CAD build for the part. Positions are in the model's coordinates, mm. Face numbers are marked on the shaded views. A direction names the side the tool comes from. Coordinates: 2 decimals unless noted, no trailing zeros. Order: outer loops, then holes, each group sorted by start corner. A loop starts at its lowest first (then second) coordinate and runs counter-clockwise, first axis right, second up. Notation, with made-up numbers: (89, 55) - (135, 55) arc R19 ccw to (135, 75) - close; hole circle Ø1 at (36.25, 0). An arc over 180 degrees is marked (long way). Write each question's results on one line, items separated by ' | '. Start each with the question number.
Q1. Pull direction Z, two halves, no side cores. Call the marked faces 1, 2 and 3: released by +Z, released by -Z, zero draft, split by the parting line, or undercut.
Q2. Band-saw the part on B-B, the plane z = -31. Write the cut outline in (x, y), then the cut area to 3 significant figures.
Q3. Band-saw the part on D-D, the plane z = 47.5. Write the cut outline in (x, y), then the cut area to 3 significant figures.
Q4. Band-saw the part on A-A, the plane z = -3. Write the cut outline in (x, y), then the cut area to 3 significant figures.
Q5. Wall check: probe 1 along X at (y, z) = (30, -5); probe 2 along X at (y, z) = (32, -34.5); probe 3 along X at (y, z) = (32, -73). Give the ranges that are in metal, low to high.
Q6. Which spindle directions (+Z, -Z, +X, -X, +Y, -Y) get a long thin tool onto all of the face, cutting with end or side? Do the marked faces 4, 5, 6, 7 and 8. Say none if no direction does.
Q7. Band-saw the part on C-C, the plane x = 140. Write the cut outline in (y, z), then the cut area to 3 significant figures.
Q8. Pin check, flat tips, straight feed: P1, Ø8, axis at x = 161, z = -59, coming from the -Y side; P2, Ø24, axis at x = 13.5, y = 31, coming from the +Z side; P3, Ø19, axis at x = 28.64, y = 30, coming from the -Z side. Stop position of each tip, or through.
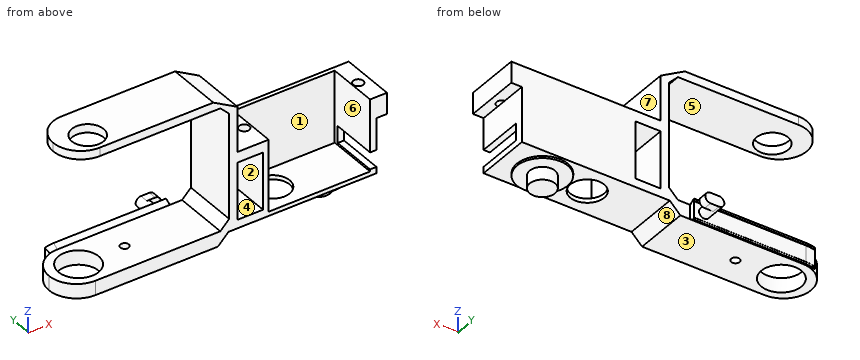
```python
from build123d import *

# Parameters (mm, degrees)
BOSS_EXTRUDE1_DEPTH = 65
BOSS_EXTRUDE2_DEPTH = 65
SKETCH5_W           = 30
SKETCH5_H           = 67.5
CUT_EXTRUDE1_DEPTH  = 65
SKETCH7_W           = 120
SKETCH7_H           = 85
CUT_EXTRUDE2_DEPTH  = 60
CUT_EXTRUDE3_REACH  = 236.375
SKETCH8_R           = 6
FILLET1_R           = 32.5
SKETCH9_R           = 18.75
CUT_EXTRUDE4_DEPTH  = 10
CUT_EXTRUDE5_START  = -17
SKETCH10_R          = 23.75
SKETCH10_R_2        = 5
CUT_EXTRUDE5_DEPTH  = 17
SKETCH11_W          = 20
SKETCH11_H          = 55
CUT_EXTRUDE6_DEPTH  = 20
SKETCH12_R          = 20
CUT_EXTRUDE7_DEPTH  = 5
SKETCH13_R          = 30
BOSS_EXTRUDE3_DEPTH = 2.5
SKETCH14_R          = 15
BOSS_EXTRUDE4_DEPTH = 15
SKETCH17_R          = 6.25
BOSS_EXTRUDE5_DEPTH = 15
BOSS_EXTRUDE6_DEPTH = 10


with BuildPart() as part:
    # Sketch2 → Boss-Extrude1 (new body)
    with BuildSketch(Plane(origin=(0, 0, 0), x_dir=(1, 0, 0), z_dir=(0, 1, 0))):
        Polygon((0, 66.142135624), (0, -66.142135624), (-28.698430784, -82.5), (-195.5, -82.5), (-195.5, -72.5), (-20.5, -72.5), (-10, -62), (-10, 62), (-20.5, 72.5), (-200.5, 72.5), (-200.5, 89.5), (-23.357864376, 89.5), align=None)
    extrude(amount=BOSS_EXTRUDE1_DEPTH)

    # Sketch3 → Boss-Extrude2 (add)
    with BuildSketch(Plane(origin=(0, 0, 0), x_dir=(1, 0, 0), z_dir=(0, 1, 0))):
        Polygon((164.142135624, 77), (164.142135624, 12), (176.642135624, 12), (176.642135624, -13), (0, -13), (0, 66.142135624), (-10.857864376, 77), align=None)
    extrude(amount=BOSS_EXTRUDE2_DEPTH)

    # Sketch5 → Cut-Extrude1 (cut)
    with BuildSketch(Plane(origin=(0, 0, 0), x_dir=(-1, 0, 0), z_dir=(0, -1, 0))):
        with Locations((-15, 33.25)):
            Rectangle(SKETCH5_W, SKETCH5_H)
    extrude(amount=-CUT_EXTRUDE1_DEPTH, mode=Mode.SUBTRACT)

    # Sketch7 → Cut-Extrude2 (cut)
    with BuildSketch(Plane(origin=(0, 0, 0), x_dir=(-1, 0, 0), z_dir=(0, -1, 0))):
        with Locations((-96.642135624, 29.5)):
            Rectangle(SKETCH7_W, SKETCH7_H)
    extrude(amount=-CUT_EXTRUDE2_DEPTH, mode=Mode.SUBTRACT)

    # Cut-Extrude3: up to this face of the body (flat: up to its plane)
    cut_extrude3_end = Plane(part.part.faces().sort_by_distance((170.392135624, 32.5, -12))[0])
    # Sketch8 → Cut-Extrude3 (cut, up to the picked face)
    with BuildSketch(Plane.XY.offset(13), mode=Mode.PRIVATE) as cut_extrude3_sk1:
        with Locations((28.642135624, 30)):
            Circle(SKETCH8_R)
    cut_extrude3_tool1 = split(extrude(cut_extrude3_sk1.sketch, amount=-CUT_EXTRUDE3_REACH, mode=Mode.PRIVATE), bisect_by=cut_extrude3_end, keep=Keep.BOTH, mode=Mode.PRIVATE)
    # Sketch8 → Cut-Extrude3 (cut, up to the picked face)
    with BuildSketch(Plane.XY.offset(13), mode=Mode.PRIVATE) as cut_extrude3_sk2:
        with Locations((163.592135624, 30)):
            Circle(SKETCH8_R)
    cut_extrude3_tool2 = split(extrude(cut_extrude3_sk2.sketch, amount=-CUT_EXTRUDE3_REACH, mode=Mode.PRIVATE), bisect_by=cut_extrude3_end, keep=Keep.BOTH, mode=Mode.PRIVATE)
    add(cut_extrude3_tool1.solids().sort_by(Axis((28.642136, 30, 13), (0, 0, -1)))[0], mode=Mode.SUBTRACT)
    add(cut_extrude3_tool2.solids().sort_by(Axis((163.592136, 30, 13), (0, 0, -1)))[0], mode=Mode.SUBTRACT)

    # Fillet1
    fillet1_edges = [part.edges().sort_by_distance(p)[0] for p in [
        (-195.5, 65, 77.5),
        (-195.5, 0, 77.5),
        (-200.5, 0, -81),
        (-200.5, 65, -81),
    ]]
    fillet(fillet1_edges, radius=FILLET1_R - 0.0001)  # a hair under: the kernel refuses the full size

    # Sketch9 → Cut-Extrude4 (cut)
    with BuildSketch(Plane.XY.offset(82.5)):
        with Locations((-160.5, 24.2)):
            Circle(SKETCH9_R)
    extrude(amount=-CUT_EXTRUDE4_DEPTH, mode=Mode.SUBTRACT)

    # Sketch10 → Cut-Extrude5 (cut)
    with BuildSketch(Plane(origin=(0, 0, -89.5), x_dir=(-1, 0, 0), z_dir=(0, 0, -1)).offset(CUT_EXTRUDE5_START)):
        with Locations((165.5, 32.5)):
            Circle(SKETCH10_R)
        with Locations((111.08276356, 32.5)):
            Circle(SKETCH10_R_2)
    extrude(amount=CUT_EXTRUDE5_DEPTH, mode=Mode.SUBTRACT)

    # Sketch11 → Cut-Extrude6 (cut)
    with BuildSketch(Plane(origin=(176.642135624, 0, 0), x_dir=(0, 0, -1), z_dir=(1, 0, 0))):
        with Locations((59.5, 27.5)):
            Rectangle(SKETCH11_W, SKETCH11_H)
    extrude(amount=-CUT_EXTRUDE6_DEPTH, mode=Mode.SUBTRACT)

    # Sketch12 → Cut-Extrude7 (cut)
    with BuildSketch(Plane(origin=(0, 0, -77), x_dir=(-1, 0, 0), z_dir=(0, 0, -1))):
        with Locations((-64.142135624, 32.5)):
            Circle(SKETCH12_R)
    extrude(amount=-CUT_EXTRUDE7_DEPTH, mode=Mode.SUBTRACT)

    # Sketch13 → Boss-Extrude3 (add)
    with BuildSketch(Plane(origin=(0, 0, -77), x_dir=(-1, 0, 0), z_dir=(0, 0, -1))):
        with Locations(Location((-117.036013704, 32.225, 0), (0, 0, 180))):
            Circle(SKETCH13_R)
    extrude(amount=BOSS_EXTRUDE3_DEPTH)

    # Sketch14 → Boss-Extrude4 (add)
    with BuildSketch(Plane(origin=(0, 0, -79.5), x_dir=(-1, 0, 0), z_dir=(0, 0, -1))):
        with Locations((-117.036013704, 32.225)):
            Circle(SKETCH14_R)
    extrude(amount=BOSS_EXTRUDE4_DEPTH)

    # Sweep1: sweep along a path in Sketch16
    with BuildLine(Plane(origin=(0, 0, 72.5), x_dir=(-1, 0, 0), z_dir=(0, 0, -1))) as sweep1_path:
        Line((35, 65), (168, 65))
        ThreePointArc((168, 65), (173, 64.613081447), (177.880948137, 63.461538462))
    # Sketch15 → Sweep1 (sweep)
    with BuildSketch(Plane.ZY.offset(35)):
        Polygon((-89.5, 65), (-72.5, 65), (-68.5, 71.278742308), (-71, 71.278742308), (-71.398085272, 71), (-90.601914728, 71), (-91, 71.278742308), (-93.5, 71.278742308), align=None)
    sweep(path=sweep1_path.line)

    # Sketch17 → Boss-Extrude5 (add)
    with BuildSketch(Plane(origin=(0, 71, 0), x_dir=(1, 0, 0), z_dir=(0, 1, 0))):
        with Locations(Location((-47.5, 81, 0), (0, 0, 270))):
            Circle(SKETCH17_R)
    extrude(amount=BOSS_EXTRUDE5_DEPTH)

    # Sketch18 → Boss-Extrude6 (add)
    with BuildSketch(Plane(origin=(0, 86, 0), x_dir=(1, 0, 0), z_dir=(0, 1, 0))):
        with BuildLine():
            Line((-47.5, 87.25), (-37.5, 87.25))
            ThreePointArc((-37.5, 87.25), (-31.25, 81), (-37.5, 74.75))
            Line((-37.5, 74.75), (-47.5, 74.75))
            ThreePointArc((-47.5, 74.75), (-53.75, 81), (-47.5, 87.25))
        make_face()
    extrude(amount=BOSS_EXTRUDE6_DEPTH)


solid = part.part
```
Results below:
1) face 1: zero draft | face 2: undercut | face 3: released by -Z
2) outline: (-10, 0) - (0, 0) - (0, 65) - (-10, 65) - close; (30, 0) - (36.64, 0) - (36.64, 60) - (156.64, 60) - (156.64, 0) - (164.14, 0) - (164.14, 65) - (30, 65) - close | area: 2,170 mm²
3) outline: (-10, 0) - (0, 0) - (0, 65) - (-10, 65) - close | area: 650 mm²
4) outline: (-10, 0) - (0, 0) - (0, 65) - (-10, 65) - close; (30, 0) - (36.64, 0) - (36.64, 60) - (156.64, 60) - (156.64, 0) - (176.64, 0) - (176.64, 65) - (30, 65) - (30, 35.84) arc R6 cw to (30, 24.16) - close; hole circle Ø12 at (163.59, 30) | area: 2,830 mm²
5) probe 1: x = -10 to 0, 34.64 to 36.64, 156.64 to 157.59, 169.59 to 176.64 | probe 2: x = -10 to 0, 30 to 36.64, 156.64 to 164.14 | probe 3: x = -200.5 to -189.24, -141.76 to -116.06, -106.11 to 44.15, 84.14 to 164.14
6) face 4: +Y, -Y | face 5: -X, +Y, -Y | face 6: +Z, -Y | face 7: +Z, +X, +Y, -Y | face 8: -Z, +Y, -Y
7) outline: (0, -77) - (12.92, -77) - (12.92, -79.5) - (51.53, -79.5) - (51.53, -77) - (65, -77) - (65, 13) - (60, 13) - (60, -72) - (0, -72) - close | area: 847 mm²
8) P1: stops at y = 55 | P2: stops at z = 13 | P3: stops at z = -77
